```python
from build123d import *

# Parameters (mm, degrees)
F1_DEPTH = 12.5
F2_W     = 8
F2_H     = 1
F2_H_2   = 1.3
F3_DEPTH = 2.301
F4_W     = 8
F4_H     = 0.8
F4_H_2   = 1.117703
F5_DEPTH = 10.001
F6_R     = 3


with BuildPart() as f1:
    # F0 (on Right) → F1 (new body, symmetric)
    with BuildSketch(Plane.YZ):
        with BuildLine():
            Line((2.3, -7), (2.3, 0))
            Line((2.3, 0), (0, 0))
            ThreePointArc((0, 0), (-1, -1), (0, -2))
            Line((0, -2), (0, -10))
            Line((0, -10), (0.8, -10))
            Line((0.8, -10), (0.8, -1))
            Line((0.8, -1), (1.5, -1))
            Line((1.5, -1), (1.5, -7))
            Line((1.5, -7), (2.3, -7))
        make_face()
    extrude(amount=F1_DEPTH, both=True)

    # F2 (on Front) → F3 (cut, through all)
    with BuildSketch(Plane.XZ):
        with Locations((0, -0.5)):
            Rectangle(F2_W, F2_H)
        with Locations((0, -9.35)):
            Rectangle(F2_W, F2_H_2)
    extrude(amount=-F3_DEPTH, mode=Mode.SUBTRACT)

    # F4 (on Top) → F5 (cut, through all)
    with BuildSketch(Plane.XY):
        with Locations((0, 1.9)):
            Rectangle(F4_W, F4_H)
        with Locations((0, -0.558851)):
            Rectangle(F4_W, F4_H_2)
    extrude(amount=-F5_DEPTH, mode=Mode.SUBTRACT)

    # F6
    f6_edges = [f1.edges().sort_by_distance(p)[0] for p in [
        (8.25, 0, -2),
        (-8.25, 0, -2),
    ]]
    fillet(f6_edges, radius=F6_R)


solid = f1.part
```
Source: CAD feature listing. Evaluate the final solid. Frame: model axes, mm. A direction names the side the tool comes from. Round coordinates to 2 decimals unless told otherwise and drop trailing zeros. Loops run counter-clockwise (first coordinate to the right, second up) from the corner with the lowest first, then second, coordinate; pieces in that order, holes last. Notation, with made-up numbers: M 81.5,36.25 L 108.5,36.25 A21 cw 108.5,55.25 Z; hole C 65.25,-33.5 d7. An arc over 180 degrees is marked long. Use a Markdown table: item, result. Add a question column.
1. Ray query, line 1 along Y through (x, z) = (-10.75, -3.75); line 2 along X through (y, z) = (1.75, -6.5); line 3 along Y through (x, z) = (9.25, -8.75). Return the intervals inside material, ascending. Write a range as [from, to].
2. Cut plane D-D, the plane y = -0.4. Output: boundary loops of the cut face in (x, z), and give its area (3 significant figures).
3. Pull-direction query (Y, two-part tool) for faces 5 (the flat face through (-8, 1.5, -4)), 6 (the flat face through (0, 0.8, -6)), 7 (the cylindrical face through (-8.19, -0.2, -2.57)), 8 (the flat face through (12.5, 0.6, -3.8)); classes: +Y half, -Y half, draft (parallel to the pull), parting line (faces both ways), or undercut.
4. Cut plane A-A, the plane y = 1.2. Output: boundary loops of the cut face in (x, z), and give its area (3 significant figures).
5. Cut plane C-C, the plane z = -7.5. Output: boundary loops of the cut face in (x, y), and give its area (3 significant figures).
6. Contact query for flat-ended pins moving along their axis: pin 1 (6 mm diameter, centred on x = -1.5, z = -4, fed in from -Y); pin 2 (5 mm diameter, centred on x = -8, z = -7, fed in from -Y). Output: stop coordinate, or through.
7. Cut plane B-B, the plane x = -8.25. Output: boundary loops of the cut face in (y, z).
8. Set-up query: faces 1 (the flat face through (8, 0, -7)), 2 (the flat face through (0, 0, -5)), 3 (the flat face through (8, 1.5, -4)), 4 (the flat face through (8, 2.3, -4)). Return all of +Z, -Z, +X, -X, +Y, -Y with unobstructed straight access to the full face (end or side cutting, diameter ignored); none if empty.
Solution:
| question | item | result |
|---|---|---|
| 1 | line 1 | y = [0, 0.8], [1.5, 2.3] |
| 1 | line 2 | x = [-12.5, -4], [4, 12.5] |
| 1 | line 3 | y = [0, 0.8] |
| 2 | outline | M -12.5,-2.15 L -4,-2.15 L -4,-0.08 L -12.5,-0.08 Z; M 4,-2.15 L 12.5,-2.15 L 12.5,-0.08 L 4,-0.08 Z |
| 2 | area | 35.1 mm2 |
| 3 | face 5 | undercut |
| 3 | face 6 | undercut |
| 3 | face 7 | -Y half |
| 3 | face 8 | draft |
| 4 | outline | M -12.5,-1 L -4,-1 L -4,0 L -12.5,0 Z; M 4,-1 L 12.5,-1 L 12.5,0 L 4,0 Z |
| 4 | area | 17.0 mm2 |
| 5 | outline | M -12.5,0 L 12.5,0 L 12.5,0.8 L -12.5,0.8 Z |
| 5 | area | 20.0 mm2 |
| 6 | pin 1 | stops at y = -0.3 |
| 6 | pin 2 | stops at y = 0 |
| 7 | outline | M -0.75,-1.66 A3 cw 0,-3.65 L 0,-10 L 0.8,-10 L 0.8,-1 L 1.5,-1 L 1.5,-7 L 2.3,-7 L 2.3,0 L 0,0 A1 ccw Z |
| 8 | face 1 | -Z, +X, -X, -Y |
| 8 | face 2 | +Z, -Z, -Y |
| 8 | face 3 | -Z, +X, -X |
| 8 | face 4 | +Z, -Z, +X, -X, +Y |
